```python
from build123d import *
from OCP.BRepFilletAPI import BRepFilletAPI_MakeChamfer

# Parameters (mm, degrees)
BOSS_EXTRUDE1_DEPTH = 19.05
CHAMFER1_SIZE       = 25.4
CHAMFER1_SIZE2      = 23.3906272
HOLE5_D             = 3.175
HOLE5_DEPTH         = 38.1
HOLE5_CSINK_D       = 10.16
HOLE5_CSINK_ANGLE   = 82
HOLE5_TIP           = 0.953866233
HOLE6_D             = 3.175
HOLE6_DEPTH         = 38.1
HOLE6_CSINK_D       = 10.16
HOLE6_CSINK_ANGLE   = 82
HOLE6_TIP           = 0.953866233


with BuildPart() as part:
    # Sketch1 → Boss-Extrude1 (new body)
    with BuildSketch(Plane.XY):
        with BuildLine():
            Line((12.7, 12.7), (12.7, -415.185594934))
            ThreePointArc((12.7, -415.185594934), (27.339445595, -436.32629993), (2.687239133, -443.641454859))
            Line((2.687239133, -443.641454859), (-518.461959982, -601.369999539))
            Line((-518.461959982, -601.369999539), (-489.829069295, -695.97562771))
            Line((-489.829069295, -695.97562771), (107.818813597, -515.094354248))
            Line((107.818813597, -515.094354248), (155.492294041, 12.7))
            Line((155.492294041, 12.7), (12.7, 12.7))
        make_face()
    extrude(amount=-BOSS_EXTRUDE1_DEPTH)

    # Chamfer1: one chamfer whose edges measure the first distance from different faces: ONE call of the kernel's chamfer builder (chamfer() names one face for all edges)
    chamfer1_edges_1 = [part.edges().sort_by_distance(p)[0] for p in [
        (155.492294041, 12.7, -9.525),
    ]]
    chamfer1_side_1 = [part.faces().sort_by_distance(p)[0] for p in [
        (84.09614702, 12.7, -9.525),
    ]]
    chamfer1_edges_2 = [part.edges().sort_by_distance(p)[0] for p in [
        (-489.829069295, -695.97562771, -9.525),
    ]]
    chamfer1 = BRepFilletAPI_MakeChamfer(part.part.solid().wrapped)
    for e in chamfer1_edges_1:
        chamfer1.Add(CHAMFER1_SIZE, CHAMFER1_SIZE2, e.wrapped, chamfer1_side_1[0].wrapped)  # the first distance lies on this face
    for e in chamfer1_edges_2:
        chamfer1.Add(CHAMFER1_SIZE, e.wrapped)
    add(Compound.cast(chamfer1.Shape()), mode=Mode.REPLACE)

    # Hole5
    with Locations(Plane(origin=(155.286738577, 10.424290059, -19.05), x_dir=(-0.08995962873759064, -0.9959454127598535, 0), z_dir=(0, 0, -1))):
        with Locations((46.221112845, 113.488854888), (39.39759596, 37.945520226), (412.28786892, 80.423559293), (407.308516105, 25.297013484), (513.561319184, 161.164706775), (597.46020397, 127.267357003), (610.543339245, 159.649253123), (694.322923815, 367.011001477), (526.644454459, 193.546602895), (610.424039029, 400.908351249)):
            CounterSinkHole(HOLE5_D / 2, HOLE5_CSINK_D / 2, depth=HOLE5_DEPTH, counter_sink_angle=HOLE5_CSINK_ANGLE)
            with Locations((0, 0, -(HOLE5_DEPTH + HOLE5_TIP / 2))):  # 118° drill point
                Cone(0, HOLE5_D / 2, HOLE5_TIP, mode=Mode.SUBTRACT)

    # Hole6
    with Locations(Plane(origin=(-643.705760022, -231.394989772, 165.474999994), x_dir=(0, 0, -1), z_dir=(-0.9571239768071421, -0.2896786029738502, -1.2569443472852944e-15))):
        with Locations((-108.649999997, 332.89193461), (108.649999997, 332.89193461), (207.774999994, 332.89193461), (174.999999994, 448.336332751), (135.266666663, 384.042401694), (176.283333328, 384.042401694), (-174.999999994, 448.336332751), (-135.266666663, 384.042401694), (-176.283333328, 384.042401694), (-207.774999994, 332.89193461)):
            CounterSinkHole(HOLE6_D / 2, HOLE6_CSINK_D / 2, depth=HOLE6_DEPTH, counter_sink_angle=HOLE6_CSINK_ANGLE)
            with Locations((0, 0, -(HOLE6_DEPTH + HOLE6_TIP / 2))):  # 118° drill point
                Cone(0, HOLE6_D / 2, HOLE6_TIP, mode=Mode.SUBTRACT)


solid = part.part
```
Geometry: final body of the model. Coordinates: model frame, mm. A direction names the side the tool comes from. Round coordinates to 2 decimals unless told otherwise and drop trailing zeros. Order: outer loops, then holes, each group sorted by start corner. A loop starts at its lowest first (then second) coordinate and runs counter-clockwise, first axis right, second up. Notation, with made-up numbers: M 4,-23.75 L 9,-23.75 A24 ccw 9,-3.75 Z; hole C -23,71.5 d5. An arc over 180 degrees is marked long. One line per item, written item: value.
(1) Cut plane C-C (x = -190.5). Return the cut outline in (y, z).
Result sheet:
outline: M -605.38,-19.05 L -502.11,-19.05 L -502.11,0 L -605.38,0 Z
(2) Pin query (flat end, axial travel): P1, Ø6, axis at y = -182.5, z = -10.5, coming from the -X side; P2, Ø8, axis at x = -335, z = -4, coming from the +Y side; P3, Ø2.5, axis at x = 93.45, y = -392.96, coming from the -Z side; P4, Ø3.5, axis at x = -84.85, y = -496.67, coming from the -Z side. Return the tip coordinate at first contact, or that it passes through.
Result sheet:
P1: x = 12.7
P2: y = -544.63
P3: through
P4: z = -15.22
(3) Cut plane A-A (z = -3.75). Give the number of separate pieces and of enclosed holes in the cut face, and give its area (3 significant figures).
Result sheet:
separate pieces: 1
enclosed holes: 7
area: 116,000 mm2
(4) Cut plane B-B (y = -294). Return the cut outline in (x, z).
Result sheet:
outline: M 12.7,-19.05 L 127.79,-19.05 L 127.79,0 L 12.7,0 Z
(5) Pull-direction query (Y, two-part tool) for faces 3 (the cylindrical face through (27.473, -435.929, -9.392)), 4 (the flat face through (-60, -466, 0)), 5 (the flat face through (-254.24, -521.4, -9.39)); classes: pulls with the +Y half, pulls with the -Y half, needs draft (parallel to the pull), parting line crosses it, or undercut.
Result sheet:
face 3: undercut
face 4: needs draft
face 5: pulls with the +Y half
(6) Line query: probe 1 along Y at (x, z) = (38.1, -11.5); probe 2 along X at (y, z) = (-25.4, -11); probe 3 along Y at (x, z) = (27, -9.25). Output: solid intervals per line, ascending. Write a range as [from, to].
Result sheet:
probe 1: [-536.2, -394.54], [-391.37, -26.99], [-23.81, 12.7]
probe 2: [12.7, 36.51], [39.69, 112.36], [115.54, 152.05]
probe 3: [-539.55, -437.21], [-424.91, 12.7]
(7) Reachability of faces 1 (the flat face through (12.7, -198, -9)), 2 (the flat face through (-182.86, -603.07, -9.39)) from +Z, -Z, +X, -X, +Y, -Y: full face, straight path, thin tool, end or side. Return the list, or none.
Result sheet:
face 1: +Z, -Z, -X, +Y
face 2: +Z, -Z, +X, -Y
